Autodesk Inventor part; units mm, degrees
ref_plane "YZ Plane" through (0, 0, 0) normal (1, 0, 0) x (0, 1, 0)
ref_plane "XZ Plane" through (0, 0, 0) normal (0, 1, 0) x (-1, 0, 0)
ref_plane "XY Plane" through (0, 0, 0) normal (0, 0, 1) x (1, 0, 0)
sketch "Sketch1" plane through (0, 0, 0) normal (0, 0, 1) x (1, 0, 0)
  line L0 (-10, -10) -> (10, -10)
  line L1 (10, -10) -> (10, 10)
  line L2 (10, 10) -> (-10, 10)
  line L3 (-10, 10) -> (-10, -10)
  line L4 (-10, -10) -> (10, 10) construction
  line L5 (10, -10) -> (-10, 10) construction
  arc A0 (2, 10) -> (-2, 10) centre (0, 10) ccw
  arc A1 (-2, -10) -> (2, -10) centre (0, -10) ccw
  point P0 (0, 0)
  dimension "d0" = 20
  dimension "d1" = 20
  dimension "d4" = 4
  dimension "d5" = 4
extrude "Extrusion1" add sketch "Sketch1" along normal blind 1.5
sketch "Sketch2" plane through (0, 0, 1.5) normal (0, 0, 1) x (1, 0, 0)
  arc A0 (2, 10) -> (-2, 10) centre (0, 10) ccw
  point P0 (0, 0)
hole "Hole1" at (0, 10, 1.5) direction (0, 0, -1) diameter 2 end through all
mirror "Mirror1" about plane through (0, 0, 0) normal (0, 1, 0) of "Hole1"
sketch "Sketch3" plane through (0, 0, 1.5) normal (0, 0, 1) x (1, 0, 0)
  line L0 (1, -5) -> (7.5, -5)
  line L1 (7.5, -5) -> (7.5, 5)
  line L2 (7.5, 5) -> (1, 5)
  line L3 (1, 5) -> (1, -5)
  line L4 (1, -5) -> (7.5, 5) construction
  line L5 (7.5, -5) -> (1, 5) construction
  circle A0 centre (0, 10) radius 1
  line L6 (1, 10) -> (1, 0) construction
  circle A1 centre (0, 10) radius 1
  line L7 (10, -10) -> (10, 10)
  line L8 (-14, 0) -> (14, 0)
  point P0 (0, 0)
  point P1 (4.25, 0)
  point P2 (4.25, 0)
  dimension "d13" = 2.5
  dimension "d14" = 10
extrude "Extrusion2" add sketch "Sketch3" along normal blind 7 contours L3 L8 L1 L0 | L3 L2 L1 L8
sketch "Sketch4" plane through (0, 0, 8.5) normal (0, 0, 1) x (1, 0, 0)
  circle A0 centre (4.25, 0) radius 2.5
  line L0 (-14, 0) -> (14, 0)
  line L1 (7.5, 5) -> (1, 5)
  line L2 (4.25, 5) -> (4.25, 0) construction
  point P0 (0, 0)
  dimension "d17" = 5
extrude "Extrusion3" add sketch "Sketch4" along normal blind 1.5
sketch "Sketch5" plane through (0, 0, 1.5) normal (0, 0, 1) x (1, 0, 0)
  line L0 (-9, 6) -> (-2, 6)
  line L1 (-2, 6) -> (-2, -6)
  line L2 (-2, -6) -> (-9, -6)
  line L3 (-9, -6) -> (-9, 6)
  line L4 (-9, 6) -> (-2, -6) construction
  line L5 (-2, 6) -> (-9, -6) construction
  line L6 (-26.8178, 0) -> (16.1363, 0)
  line L7 (-10, 10) -> (-10, -10)
  point P0 (0, 0)
  point P1 (-5.5, 0)
  point P2 (-5.5, 0)
  dimension "d20" = 7
  dimension "d21" = 12
  dimension "d22" = 1
extrude "Extrusion4" add sketch "Sketch5" along normal blind 8.5
properties part number "button"
Can you work these out from the model? Positions are in its coordinate system, mm. A direction names the side the tool comes from. Coordinates: 2 decimals unless noted, no trailing zeros. Write each loop counter-clockwise with the first axis right and the second up, starting at its lowest first coordinate (ties: lowest second). Pieces come first, ordered by that corner, then holes. Notation, with made-up numbers: (39, 7) - (94, 7) arc R31 cw to (94, 31) - close; hole circle Ø8 at (49.25, -16.75). An arc over 180 degrees is marked (long way). Return JSON: item names as keys, results as strings.
Q1. I'm going to push flat-ended pins straight in: pin 1 Ø2.5 at (y, z) = (-1, 6) entering from -X; pin 2 Ø1.2 at (x, z) = (4.5, 0.5) entering from -Y; pin 3 Ø1 at (y, z) = (-8, 6) entering from -X; pin 4 Ø2.5 at (x, y) = (0, 10) entering from +Z. Where does each tip first touch, or does it pass through?
Computed values:
{"pin 1": "stops at x = -9", "pin 2": "stops at y = -10", "pin 3": "passes through", "pin 4": "stops at z = 1.5"}
Q2. Thinking about a two-plate mould opening in X: for faces 6 (the cylindrical face through (6.635, -0.751, 9.24)), 7 (the flat face through (-9, 0, 6)), 8 (the flat face through (2.8, 2.3, 8.5)), 9 (the flat face through (4, 0, 10)), which applies, +X half, -X half, draft (parallel to the pull), parting line (faces both ways), or undercut?
Computed values:
{"face 6": "undercut", "face 7": "-X half", "face 8": "undercut", "face 9": "draft"}
Q3. If we section it at A-A (z = 0.75): Please give me the cut outline in (x, y).
Computed values:
{"outline": "(-10, -10) - (-2, -10) arc R2 ccw to (2, -10) - (10, -10) - (10, 10) - (2, 10) arc R2 ccw to (-2, 10) - (-10, 10) - close; hole circle Ø2 at (0, -10); hole circle Ø2 at (0, 10)"}
Q4. If we section it at D-D (y = 3.25): Please give me the cut outline in (x, z).
Computed values:
{"outline": "(-10, 0) - (10, 0) - (10, 1.5) - (7.5, 1.5) - (7.5, 8.5) - (1, 8.5) - (1, 1.5) - (-2, 1.5) - (-2, 10) - (-9, 10) - (-9, 1.5) - (-10, 1.5) - close"}
Q5. If we section it at B-B (z = 5.5): Please give me the cut outline in (x, y).
Computed values:
{"outline": "(-9, -6) - (-2, -6) - (-2, 6) - (-9, 6) - close; (1, -5) - (7.5, -5) - (7.5, 5) - (1, 5) - close"}
Q6. Please list where these lines run through material, in increasing order: L1, parallel to Y at x = 0, z = 0.4; L2, parallel to X at y = -3.5, z = 3.5; L3, parallel to Z at x = 4.5, y = 9.5. Write a range as from..to.
Computed values:
{"L1": "y = -12..-11, -9..9, 11..12", "L2": "x = -9..-2, 1..7.5", "L3": "z = 0..1.5"}
Q7. If we section it at C-C (x = 0): Please give me the cut outline in (y, z), then the cut area to 3 significant figures.
Computed values:
{"outline": "(-12, 0) - (-11, 0) - (-11, 1.5) - (-12, 1.5) - close; (-9, 0) - (9, 0) - (9, 1.5) - (-9, 1.5) - close; (11, 0) - (12, 0) - (12, 1.5) - (11, 1.5) - close", "area": "30.0 mm2"}
Q8. On a 3-axis mill with a long thin cutter (end or side, diameter ignored), from which of +Z, -Z, +X, -X, +Y, -Y can I reach the whole of each face in a straight line? I mean faces 1 (the flat face through (7.5, 0, 5)), 2 (the flat face through (-6, 10, 1)), 3 (the flat face through (1, 0, 5)), 4 (the flat face through (6, -10, 1)), 5 (the flat face through (-5, -6, 6)). Say none if no direction works.
Computed values:
{"face 1": "+Z, +X, +Y, -Y", "face 2": "+Z, -Z, -X, +Y", "face 3": "+Z, +Y, -Y", "face 4": "+Z, -Z, +X, -Y", "face 5": "+Z, +X, -X, -Y"}
